```python
from build123d import *

# Parameters (mm, degrees)
BOSS_EXTRUDE1_DEPTH = 33.02
CUT_EXTRUDE1_DEPTH  = 25.4
SKETCH3_R           = 3.175
CUT_EXTRUDE2_DEPTH  = 34.02
SKETCH4_R           = 5.715
CUT_EXTRUDE3_DEPTH  = 3.81


with BuildPart() as part:
    # Sketch1 → Boss-Extrude1 (new body)
    with BuildSketch(Plane(origin=(0, 0, 0), x_dir=(1, 0, 0), z_dir=(0, 1, 0))):
        with BuildLine():
            Line((-63.5, -50.8), (63.5, -50.8))
            ThreePointArc((63.5, -50.8), (72.480256121, -47.080256121), (76.2, -38.1))
            Line((76.2, -38.1), (76.2, 38.1))
            ThreePointArc((76.2, 38.1), (72.480256121, 47.080256121), (63.5, 50.8))
            Line((63.5, 50.8), (-63.5, 50.8))
            ThreePointArc((-63.5, 50.8), (-72.480256121, 47.080256121), (-76.2, 38.1))
            Line((-76.2, 38.1), (-76.2, -38.1))
            ThreePointArc((-76.2, -38.1), (-72.480256121, -47.080256121), (-63.5, -50.8))
        make_face()
    extrude(amount=BOSS_EXTRUDE1_DEPTH)

    # Sketch2 → Cut-Extrude1 (cut)
    with BuildSketch(Plane(origin=(0, 33.02, 0), x_dir=(1, 0, 0), z_dir=(0, 1, 0))):
        with BuildLine():
            Line((-76.2, 19.759327566), (-76.2, -24.765))
            ThreePointArc((-76.2, -24.765), (-73.518450651, -13.405774674), (-66.04, -4.445))
            Line((-66.04, -4.445), (-34.215351473, 19.423486395))
            ThreePointArc((-34.215351473, 19.423486395), (-28.356838342, 20.838097819), (-23.30312823, 17.55430189))
            Line((-23.30312823, 17.55430189), (7.241229349, -28.262234478))
            ThreePointArc((7.241229349, -28.262234478), (25.097671742, -39.864980093), (45.797751473, -34.866686395))
            Line((45.797751473, -34.866686395), (76.2, -12.065))
            Line((76.2, -12.065), (76.2, 12.065))
            Line((76.2, 12.065), (34.215351473, -19.423486395))
            ThreePointArc((34.215351473, -19.423486395), (28.356838342, -20.838097819), (23.30312823, -17.55430189))
            Line((23.30312823, -17.55430189), (-7.241229349, 28.262234478))
            ThreePointArc((-7.241229349, 28.262234478), (-25.097671742, 39.864980093), (-45.797751473, 34.866686395))
            ThreePointArc((-45.797751473, 34.866686395), (-60.308353779, 25.923391468), (-76.2, 19.759327566))
        make_face()
    extrude(amount=-CUT_EXTRUDE1_DEPTH, mode=Mode.SUBTRACT)

    # Sketch3 → Cut-Extrude2 (cut, through all)
    with BuildSketch(Plane(origin=(0, 33.02, 0), x_dir=(1, 0, 0), z_dir=(0, 1, 0))):
        with Locations((63.5, 36.83)):
            Circle(SKETCH3_R)
        with Locations((0, 36.83)):
            Circle(SKETCH3_R)
        with Locations((-63.5, 36.83)):
            Circle(SKETCH3_R)
        with Locations((63.5, -36.83)):
            Circle(SKETCH3_R)
        with Locations((0, -36.83)):
            Circle(SKETCH3_R)
        with Locations((-63.5, -36.83)):
            Circle(SKETCH3_R)
    extrude(amount=-CUT_EXTRUDE2_DEPTH, mode=Mode.SUBTRACT)

    # Sketch4 → Cut-Extrude3 (cut)
    with BuildSketch(Plane(origin=(0, 33.02, 0), x_dir=(1, 0, 0), z_dir=(0, 1, 0))):
        with Locations((-63.5, 36.83)):
            Circle(SKETCH4_R)
        with Locations((0, 36.83)):
            Circle(SKETCH4_R)
        with Locations((63.5, 36.83)):
            Circle(SKETCH4_R)
        with Locations((63.5, -36.83)):
            Circle(SKETCH4_R)
        with Locations((0, -36.83)):
            Circle(SKETCH4_R)
        with Locations((-63.5, -36.83)):
            Circle(SKETCH4_R)
    extrude(amount=-CUT_EXTRUDE3_DEPTH, mode=Mode.SUBTRACT)


solid = part.part
```
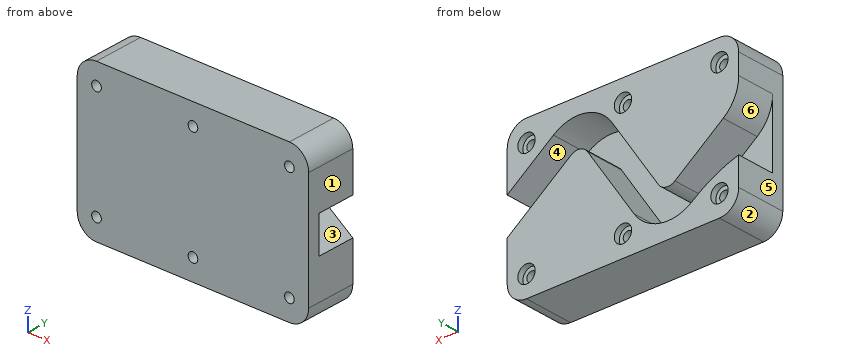
Could you check a few things on this model? Use its own coordinates, in mm. Face numbers are marked on the shaded views. A direction names the side the tool comes from. Give positions to 0.01 mm unless a question says otherwise; leave off trailing zeros. Write each loop counter-clockwise with the first axis right and the second up, starting at its lowest first coordinate (ties: lowest second). Pieces come first, ordered by that corner, then holes. Notation, with made-up numbers: (52.25, -33.5) - (103.25, -33.5) arc R19 ccw to (103.25, 1.5) - close; hole circle Ø3 at (56, 19.5). An arc over 180 degrees is marked (long way). One line per item, written item: value. Start each with the question number.
Item 1: Imagine slicing it at C-C, the plane x = 0. List the corners of the cut face in (y, z) for me (3 decimals), and give its area (3 significant figures).
Item 2: Imagine slicing it at D-D, the plane z = 8.5. List the corners of the cut face in (x, y) for me.
Item 3: Imagine slicing it at B-B, the plane y = 6. List the corners of the cut face in (x, z) for me (3 decimals).
Item 4: If we mould it in two halves opening along Z, with no side actions, what happens to the marked faces 1, 2 and 3? For each: +Z half, -Z half, draft (parallel to the pull), parting line (faces both ways), or undercut.
Item 5: Which directions (+Z, -Z, +X, -X, +Y, -Y) give clear straight access to the entire face, cutting with the end or side of a thin tool? Please do the marked faces 4, 5 and 6.
Item 6: Please list where these lines run through material, in increasing order: line 1 (X direction, y = 15, z = 36); line 2 (X direction, y = 8, z = 35); line 3 (Z direction, x = -63, y = 30) (3 decimals). Write a range as from..to.
Item 7: I'm going to push flat-ended pins straight in: pin 1 (9 mm diameter, centred on x = 63.5, z = -36.83, fed in from +Y); pin 2 (4 mm diameter, centred on x = 0, z = -36.83, fed in from +Y); pin 3 (12 mm diameter, centred on y = 15, z = -4.5, fed in from -X). Where does each tip first touch, or does it pass through?
Item 8: Imagine slicing it at A-A, the plane y = 27.5. List the corners of the cut face in (x, z) for me (3 decimals).
Geometry says:
1. outline: (0, -50.8) - (33.02, -50.8) - (33.02, -42.545) - (29.21, -42.545) - (29.21, -40.005) - (0, -40.005) - close; (0, -33.655) - (29.21, -33.655) - (29.21, -31.115) - (33.02, -31.115) - (33.02, -17.4) - (7.62, -17.4) - (7.62, 17.4) - (33.02, 17.4) - (33.02, 31.115) - (29.21, 31.115) - (29.21, 33.655) - (0, 33.655) - close; (0, 40.005) - (29.21, 40.005) - (29.21, 42.545) - (33.02, 42.545) - (33.02, 50.8) - (0, 50.8) - close
1. area: 2,010 mm^2
2. outline: (-76.2, 0) - (76.2, 0) - (76.2, 7.62) - (48.78, 7.62) - (48.78, 33.02) - (17.27, 33.02) - (17.27, 7.62) - (-5.93, 7.62) - (-5.93, 33.02) - (-70.31, 33.02) - (-70.31, 7.62) - (-76.2, 7.62) - close
3. outline: (-76.2, -38.1) arc R12.7 ccw to (-63.5, -50.8) - (63.5, -50.8) arc R12.7 ccw to (76.2, -38.1) - (76.2, 38.1) arc R12.7 ccw to (63.5, 50.8) - (-63.5, 50.8) arc R12.7 ccw to (-76.2, 38.1) - close; hole circle Ø6.35 at (-63.5, -36.83); hole circle Ø6.35 at (-63.5, 36.83); hole circle Ø6.35 at (0, -36.83); hole circle Ø6.35 at (0, 36.83); hole circle Ø6.35 at (63.5, -36.83); hole circle Ø6.35 at (63.5, 36.83)
4. face 1: draft
4. face 2: -Z half
4. face 3: undercut
5. face 4: +Y
5. face 5: +Z, -Z, -X, +Y, -Y
5. face 6: -X, +Y
6. line 1: -76.2..-66.56, -60.44..-3.06, 3.06..15.12, 44.16..60.44, 66.56..76.2
6. line 2: -76.2..-66.09, -60.91..-2.59, 2.59..13.67, 45.62..60.91, 66.09..76.2
6. line 3: -50.8..-42.523, -31.137..-24.639, 2.165..31.137, 42.523..50.8
7. pin 1: y = 29.21
7. pin 2: through
7. pin 3: x = -62.11
8. outline: (-76.2, -38.1) arc R12.7 ccw to (-63.5, -50.8) - (63.5, -50.8) arc R12.7 ccw to (76.2, -38.1) - (76.2, -12.065) - (34.215, 19.423) arc R7.62 ccw to (23.303, 17.554) - (-7.241, -28.262) arc R26.924 cw to (-45.798, -34.867) arc R93.618 ccw to (-76.2, -19.759) - close; (-76.2, 24.765) arc R25.4 ccw to (-66.04, 4.445) - (-34.215, -19.423) arc R7.62 ccw to (-23.303, -17.554) - (7.241, 28.262) arc R26.924 cw to (45.798, 34.867) - (76.2, 12.065) - (76.2, 38.1) arc R12.7 ccw to (63.5, 50.8) - (-63.5, 50.8) arc R12.7 ccw to (-76.2, 38.1) - close; hole circle Ø6.35 at (-63.5, -36.83); hole circle Ø6.35 at (-63.5, 36.83); hole circle Ø6.35 at (0, -36.83); hole circle Ø6.35 at (0, 36.83); hole circle Ø6.35 at (63.5, -36.83); hole circle Ø6.35 at (63.5, 36.83)
